Model file for the job. Use its own axes, mm. A direction names the side the tool comes from. Round coordinates to 2 decimals unless told otherwise and drop trailing zeros. Order: outer loops, then holes, each group sorted by start corner. A loop starts at its lowest first (then second) coordinate and runs counter-clockwise, first axis right, second up. Notation, with made-up numbers: (75, 1.25) - (113, 1.25) arc R25 ccw to (113, 25.25) - close; hole circle Ø10 at (-33, -1.5). An arc over 180 degrees is marked (long way). Answer as CSV lines item,"result". Start each with the question number.
1. Wall check: line 1 along X through (y, z) = (15.5, 0); line 2 along X through (y, z) = (11.25, -4); line 3 along Z through (x, y) = (-2.25, 15.25). Give the ranges that are in metal, low to high. Write a range as [from, to].
2. Band-saw the part on A-A on z = 0. List the corners of the cut face in (x, y).
3. Pull direction X, two halves, no side cores. Call faces 3 (the face through (-7, 20, 0)), 4 (the face through (-15, 10, 0)), 5 (the face through (-4.43, 10.14, 7.4)): released by +X, released by -X, zero draft, split by the parting line, or undercut.
4. 3-axis set-ups, long thin cutter, end or side, ignore diameter. For faces 1 (the face through (0, 10, -12.5)), 2 (the face through (-4.4, 10.14, -7.43)): which of +Z, -Z, +X, -X, +Y, -Y reach the whole face in a straight line?
5. Pin check, flat tips, straight feed: pin 1 Ø5 at (x, z) = (10, 0) entering from +Y; pin 2 Ø3 at (x, z) = (-10, 0) entering from +Y. Stop position of each tip, or through.
6. Band-saw the part on D-D on x = 11. List the corners of the cut face in (y, z), then the cut area to 3 significant figures.
7. Band-saw the part on B-B on x = -10. List the corners of the cut face in (y, z), then the cut area to 3 significant figures.
8. Band-saw the part on C-C on y = 16.5. List the corners of the cut face in (x, z), then the cut area to 3 significant figures.
```python
from build123d import *

# Parameters (mm, degrees)
SKETCH_1_W          = 30
SKETCH_1_H          = 25
SKETCH_1_R          = 1.6
EXTRUDE_1_DEPTH     = 20
CUT_EXTRUDE_1_DEPTH = 20


with BuildPart() as part:
    # 草图1 → 凸台-拉伸1 (new body)
    with BuildSketch(Plane(origin=(0, 0, 0), x_dir=(1, 0, 0), z_dir=(0, 1, 0))):
        Rectangle(SKETCH_1_W, SKETCH_1_H)
        with Locations(Location((-10, 0, 0), (0, 0, 270))):
            Circle(SKETCH_1_R, mode=Mode.SUBTRACT)
        with Locations(Location((10, 0, 0), (0, 0, 270))):
            Circle(SKETCH_1_R, mode=Mode.SUBTRACT)
    extrude(amount=EXTRUDE_1_DEPTH)

    # 草图2 → 切除-拉伸1 (cut)
    with BuildSketch(Plane(origin=(0, 20, 0), x_dir=(1, 0, 0), z_dir=(0, 1, 0))):
        with BuildLine():
            Line((-3, -8), (3, -8))
            ThreePointArc((3, -8), (4.414213562, -7.414213562), (5, -6))
            Line((5, -6), (5, 6))
            ThreePointArc((5, 6), (4.414213562, 7.414213562), (3, 8))
            Line((3, 8), (-3, 8))
            ThreePointArc((-3, 8), (-4.414213562, 7.414213562), (-5, 6))
            Line((-5, 6), (-5, -6))
            ThreePointArc((-5, -6), (-4.414213562, -7.414213562), (-3, -8))
        make_face()
    extrude(amount=-CUT_EXTRUDE_1_DEPTH, mode=Mode.SUBTRACT)


solid = part.part
```
Reply:
1,line 1,"x = [-15, -11.6], [-8.4, -5], [5, 8.4], [11.6, 15]"
1,line 2,"x = [-15, -5], [5, 15]"
1,line 3,"z = [-12.5, -8], [8, 12.5]"
2,outline,"(-15, 0) - (-11.6, 0) - (-11.6, 20) - (-15, 20) - close; (-8.4, 0) - (-5, 0) - (-5, 20) - (-8.4, 20) - close; (5, 0) - (8.4, 0) - (8.4, 20) - (5, 20) - close; (11.6, 0) - (15, 0) - (15, 20) - (11.6, 20) - close"
3,face 3,"zero draft"
3,face 4,"released by -X"
3,face 5,"undercut"
4,face 1,"-Z, +X, -X, +Y, -Y"
4,face 2,"+Y, -Y"
5,pin 1,"stops at y = 20"
5,pin 2,"passes through"
6,outline,"(0, -12.5) - (20, -12.5) - (20, -1.25) - (0, -1.25) - close; (0, 1.25) - (20, 1.25) - (20, 12.5) - (0, 12.5) - close"
6,area,"450 mm2"
7,outline,"(0, -12.5) - (20, -12.5) - (20, -1.6) - (0, -1.6) - close; (0, 1.6) - (20, 1.6) - (20, 12.5) - (0, 12.5) - close"
7,area,"436 mm2"
8,outline,"(-15, -12.5) - (15, -12.5) - (15, 12.5) - (-15, 12.5) - close; hole circle Ø3.2 at (-10, 0); hole (-5, -6) arc R2 ccw to (-3, -8) - (3, -8) arc R2 ccw to (5, -6) - (5, 6) arc R2 ccw to (3, 8) - (-3, 8) arc R2 ccw to (-5, 6) - close; hole circle Ø3.2 at (10, 0)"
8,area,"577 mm2"
